Could you check a few things on this model? Use its own coordinates, in mm. A direction names the side the tool comes from. Round coordinates to 2 decimals unless told otherwise and drop trailing zeros. Order: outer loops, then holes, each group sorted by start corner. A loop starts at its lowest first (then second) coordinate and runs counter-clockwise, first axis right, second up. Notation, with made-up numbers: (44.25, 46.25) -> (54.25, 46.25) arc R7 cw to (54.25, 53.25) -> close; hole circle Ø3 at (-38.75, 37). An arc over 180 degrees is marked (long way). One line per question, with ' | ' between items.
Autodesk Inventor part; units mm, degrees
ref_plane "YZ Plane" through (0, 0, 0) normal (1, 0, 0) x (0, 1, 0)
ref_plane "XZ Plane" through (0, 0, 0) normal (0, 1, 0) x (-1, 0, 0)
ref_plane "XY Plane" through (0, 0, 0) normal (0, 0, 1) x (1, 0, 0)
sketch "Sketch1" plane through (0, 0, 0) normal (0, 0, 1) x (1, 0, 0)
  line L0 (0, -42.8392) -> (0, 0.8108)
  line L1 (0, 0) -> (49.5875, 0)
  line L2 (0, -42.8392) -> (10, -42.8392)
  line L3 (10, -42.8392) -> (49.5875, -10)
  line L4 (49.5875, -10) -> (49.5875, 0)
  line L5 (0, -42.8392) -> (0, 0)
  line L6 (0, 0) -> (49.5875, 0)
  line L7 (21.7117, 0) -> (36.5117, 0) construction
  dimension "d0" = 10
  dimension "d1" = 10
extrude "Extrusion1" add sketch "Sketch1" against normal blind 4
fillet "Fillet1" radius 2 2 edges at (49.5875, -10, -2) (10, -42.8392, -2)
sketch "Sketch2" plane through (0, 0, 0) normal (0, 0, 1) x (1, 0, 0)
  line L0 (14.6536, -1.8875) -> (0, -1.8875) construction
  line L1 (0, -1.8875) -> (0, -8.7634)
  line L2 (0, -8.7634) -> (-6.35, -8.7634)
  line L3 (-6.35, -8.7634) -> (-6.35, -14.7634)
  line L4 (-6.35, -14.7634) -> (0, -14.7634)
  line L5 (0, -14.7634) -> (0, -20.8634)
  line L6 (0, -20.8634) -> (6, -20.8634)
  line L7 (6, -20.8634) -> (6, -19.6134)
  line L8 (6, -19.6134) -> (8, -19.6134)
  line L9 (8, -19.6134) -> (8, -20.8634)
  line L10 (8, -20.8634) -> (10.65, -20.8634)
  line L11 (10.65, -20.8634) -> (10.65, -23.8634)
  line L12 (10.65, -23.8634) -> (8, -23.8634)
  line L13 (8, -23.8634) -> (8, -25.1134)
  line L14 (8, -25.1134) -> (6, -25.1134)
  line L15 (6, -25.1134) -> (6, -23.8634)
  line L16 (6, -23.8634) -> (0, -23.8634)
  line L17 (0, -23.8634) -> (0, -29.9634)
  line L18 (0, -29.9634) -> (-6.35, -29.9634)
  line L19 (-6.35, -29.9634) -> (-6.35, -35.9634)
  line L20 (-6.35, -35.9634) -> (0, -35.9634)
  line L21 (0, -35.9634) -> (0, -42.8392)
  line L22 (0, -42.8392) -> (14.6536, -42.8392)
  line L23 (14.6536, -42.8392) -> (14.6536, -1.8875) construction
  line L24 (49.5875, -14.6536) -> (49.5875, 0)
  line L25 (49.5875, 0) -> (42.7117, 0)
  line L26 (42.7117, 0) -> (42.7117, 6.35)
  line L27 (42.7117, 6.35) -> (36.7117, 6.35)
  line L28 (36.7117, 6.35) -> (36.7117, 0)
  line L29 (36.7117, 0) -> (30.6117, 0)
  line L30 (30.6117, 0) -> (30.6117, -6)
  line L31 (30.6117, -6) -> (31.8617, -6)
  line L32 (31.8617, -6) -> (31.8617, -8)
  line L33 (31.8617, -8) -> (30.6117, -8)
  line L34 (30.6117, -8) -> (30.6117, -10.65)
  line L35 (30.6117, -10.65) -> (27.6117, -10.65)
  line L36 (27.6117, -10.65) -> (27.6117, -8)
  line L37 (27.6117, -8) -> (26.3617, -8)
  line L38 (26.3617, -8) -> (26.3617, -6)
  line L39 (26.3617, -6) -> (27.6117, -6)
  line L40 (27.6117, -6) -> (27.6117, 0)
  line L41 (27.6117, 0) -> (21.5117, 0)
  line L42 (21.5117, 0) -> (21.5117, 6.35)
  line L43 (21.5117, 6.35) -> (15.5117, 6.35)
  line L44 (15.5117, 6.35) -> (15.5117, 0)
  line L45 (15.5117, 0) -> (8.6359, 0)
  line L46 (8.6359, 0) -> (8.6359, -14.6536) construction
  line L47 (8.6359, -14.6536) -> (49.5875, -14.6536) construction
  line L48 (49.5875, 0) -> (0, -42.8392)
  line L49 (8.6359, 0) -> (0, -1.8875)
  point P0 (0, 0)
extrude "Extrusion2" add sketch "Sketch2" against normal blind 4
sketch "Sketch3" plane through (0, 0, 0) normal (0, 0, 1) x (1, 0, 0)
  line L0 (14.6536, -1.8875) -> (0, -1.8875)
  line L1 (0, -1.8875) -> (0, -8.7634)
  line L2 (0, -8.7634) -> (-6.35, -8.7634)
  line L3 (-6.35, -8.7634) -> (-6.35, -14.7634)
  line L4 (-6.35, -14.7634) -> (0, -14.7634)
  line L5 (0, -14.7634) -> (0, -20.8634)
  line L6 (0, -20.8634) -> (6, -20.8634)
  line L7 (6, -20.8634) -> (6, -19.6134)
  line L8 (6, -19.6134) -> (8, -19.6134)
  line L9 (8, -19.6134) -> (8, -20.8634)
  line L10 (8, -20.8634) -> (10.65, -20.8634)
  line L11 (10.65, -20.8634) -> (10.65, -23.8634)
  line L12 (10.65, -23.8634) -> (8, -23.8634)
  line L13 (8, -23.8634) -> (8, -25.1134)
  line L14 (8, -25.1134) -> (6, -25.1134)
  line L15 (6, -25.1134) -> (6, -23.8634)
  line L16 (6, -23.8634) -> (0, -23.8634)
  line L17 (0, -23.8634) -> (0, -29.9634)
  line L18 (0, -29.9634) -> (-6.35, -29.9634)
  line L19 (-6.35, -29.9634) -> (-6.35, -35.9634)
  line L20 (-6.35, -35.9634) -> (0, -35.9634)
  line L21 (0, -35.9634) -> (0, -42.8392)
  line L22 (0, -42.8392) -> (14.6536, -42.8392)
  line L23 (14.6536, -42.8392) -> (14.6536, -1.8875)
  line L24 (49.5875, -14.6536) -> (49.5875, 0)
  line L25 (49.5875, 0) -> (42.7117, 0)
  line L26 (42.7117, 0) -> (42.7117, 6.35)
  line L27 (42.7117, 6.35) -> (36.7117, 6.35)
  line L28 (36.7117, 6.35) -> (36.7117, 0)
  line L29 (36.7117, 0) -> (30.6117, 0)
  line L30 (30.6117, 0) -> (30.6117, -6)
  line L31 (30.6117, -6) -> (31.8617, -6)
  line L32 (31.8617, -6) -> (31.8617, -8)
  line L33 (31.8617, -8) -> (30.6117, -8)
  line L34 (30.6117, -8) -> (30.6117, -10.65)
  line L35 (30.6117, -10.65) -> (27.6117, -10.65)
  line L36 (27.6117, -10.65) -> (27.6117, -8)
  line L37 (27.6117, -8) -> (26.3617, -8)
  line L38 (26.3617, -8) -> (26.3617, -6)
  line L39 (26.3617, -6) -> (27.6117, -6)
  line L40 (27.6117, -6) -> (27.6117, 0)
  line L41 (27.6117, 0) -> (21.5117, 0)
  line L42 (21.5117, 0) -> (21.5117, 6.35)
  line L43 (21.5117, 6.35) -> (15.5117, 6.35)
  line L44 (15.5117, 6.35) -> (15.5117, 0)
  line L45 (15.5117, 0) -> (8.6359, 0)
  line L46 (8.6359, 0) -> (8.6359, -14.6536)
  line L47 (8.6359, -14.6536) -> (49.5875, -14.6536)
  line L48 (0, -23.8634) -> (0, -20.8634)
  line L49 (0, -14.7634) -> (0, -29.9634)
  line L50 (27.6117, 0) -> (30.6117, 0)
  line L51 (36.7117, 0) -> (21.5117, 0)
  point P0 (0, 0)
extrude "Extrusion3" cut sketch "Sketch3" against normal blind 4 contours L6 L7 L8 L9 L10 L11 L12 L13 L14 L15 L16 L48 | L50 L30 L31 L32 L33 L34 L35 L36 L37 L38 L39 L40
sketch "Sketch4" plane through (0, 0, 0) normal (0, 0, 1) x (1, 0, 0)
  line L0 (30.6117, 0) -> (30.6117, -6)
  line L1 (30.6117, -6) -> (31.8617, -6)
  line L2 (31.8617, -6) -> (31.8617, -8)
  line L3 (31.8617, -8) -> (30.6117, -8)
  line L4 (30.6117, -8) -> (30.6117, -10.65)
  line L5 (30.6117, -10.65) -> (27.6117, -10.65)
  line L6 (27.6117, -10.65) -> (27.6117, -8)
  line L7 (27.6117, -8) -> (26.3617, -8)
  line L8 (26.3617, -8) -> (26.3617, -6)
  line L9 (26.3617, -6) -> (27.6117, -6)
  line L10 (27.6117, -6) -> (27.6117, 0)
  line L11 (27.6117, 0) -> (21.5117, 0)
  line L12 (21.5117, 0) -> (21.5117, 6.35)
  line L13 (21.5117, 6.35) -> (15.5117, 6.35)
  line L14 (15.5117, 6.35) -> (15.5117, 0)
  line L15 (15.5117, 0) -> (0, 0)
  line L16 (0, 0) -> (0, -8.7634)
  line L17 (0, -8.7634) -> (-6.35, -8.7634)
  line L18 (-6.35, -8.7634) -> (-6.35, -14.7634)
  line L19 (-6.35, -14.7634) -> (0, -14.7634)
  line L20 (0, -14.7634) -> (0, -29.9634)
  line L21 (0, -29.9634) -> (-6.35, -29.9634)
  line L22 (-6.35, -29.9634) -> (-6.35, -35.9634)
  line L23 (-6.35, -35.9634) -> (0, -35.9634)
  line L24 (0, -35.9634) -> (0, -42.8392)
  line L25 (0, -42.8392) -> (9.2784, -42.8392)
  arc A0 (9.2784, -42.8392) -> (10.5554, -42.3785) centre (9.2784, -40.8392) ccw
  line L26 (10.5554, -42.3785) -> (48.8645, -10.5998)
  arc A1 (48.8645, -10.5998) -> (49.5875, -9.0605) centre (47.5875, -9.0605) ccw
  line L27 (49.5875, -9.0605) -> (49.5875, 0)
  line L28 (49.5875, 0) -> (42.7117, 0)
  line L29 (42.7117, 0) -> (42.7117, 6.35)
  line L30 (42.7117, 6.35) -> (36.7117, 6.35)
  line L31 (36.7117, 6.35) -> (36.7117, 0)
  line L32 (36.7117, 0) -> (30.6117, 0)
  line L33 (6, -23.8634) -> (0, -23.8634)
  line L34 (0, -23.8634) -> (0, -20.8634)
  line L35 (0, -20.8634) -> (6, -20.8634)
  line L36 (6, -20.8634) -> (6, -19.6134)
  line L37 (6, -19.6134) -> (8, -19.6134)
  line L38 (8, -19.6134) -> (8, -20.8634)
  line L39 (8, -20.8634) -> (10.65, -20.8634)
  line L40 (10.65, -20.8634) -> (10.65, -23.8634)
  line L41 (10.65, -23.8634) -> (8, -23.8634)
  line L42 (8, -23.8634) -> (8, -25.1134)
  line L43 (8, -25.1134) -> (6, -25.1134)
  line L44 (6, -25.1134) -> (6, -23.8634)
  line L45 (36.7117, 0) -> (30.6117, 0)
  line L46 (27.6117, 0) -> (30.6117, 0)
  line L47 (36.9117, 0) -> (36.9117, 6.15)
  line L48 (36.9117, 6.15) -> (42.5117, 6.15)
  line L49 (42.5117, 6.15) -> (42.5117, -0.2)
  line L50 (42.5117, -0.2) -> (49.3875, -0.2)
  line L51 (49.3875, -0.2) -> (49.3875, -9.0605)
  arc A2 (48.7368, -10.4459) -> (49.3875, -9.0605) centre (47.5875, -9.0605) ccw
  line L52 (48.7368, -10.4459) -> (10.4277, -42.2246)
  arc A3 (9.2784, -42.6392) -> (10.4277, -42.2246) centre (9.2784, -40.8392) ccw
  line L53 (9.2784, -42.6392) -> (0.2, -42.6392)
  line L54 (0.2, -42.6392) -> (0.2, -35.7634)
  line L55 (0.2, -35.7634) -> (-6.15, -35.7634)
  line L56 (-6.15, -35.7634) -> (-6.15, -30.1634)
  line L57 (-6.15, -30.1634) -> (0.2, -30.1634)
  line L58 (0.2, -30.1634) -> (0.2, -14.5634)
  line L59 (0.2, -14.5634) -> (-6.15, -14.5634)
  line L60 (-6.15, -14.5634) -> (-6.15, -8.9634)
  line L61 (-6.15, -8.9634) -> (0.2, -8.9634)
  line L62 (0.2, -8.9634) -> (0.2, -0.2)
  line L63 (0.2, -0.2) -> (15.7117, -0.2)
  line L64 (15.7117, -0.2) -> (15.7117, 6.15)
  line L65 (15.7117, 6.15) -> (21.3117, 6.15)
  line L66 (21.3117, 6.15) -> (21.3117, -0.2)
  line L67 (27.4117, -0.2) -> (27.4117, -5.8)
  line L68 (27.4117, -5.8) -> (26.1617, -5.8)
  line L69 (26.1617, -5.8) -> (26.1617, -8.2)
  line L70 (26.1617, -8.2) -> (27.4117, -8.2)
  line L71 (27.4117, -8.2) -> (27.4117, -10.85)
  line L72 (27.4117, -10.85) -> (30.8117, -10.85)
  line L73 (30.8117, -10.85) -> (30.8117, -8.2)
  line L74 (30.8117, -8.2) -> (32.0617, -8.2)
  line L75 (32.0617, -8.2) -> (32.0617, -5.8)
  line L76 (32.0617, -5.8) -> (30.8117, -5.8)
  line L77 (30.8117, -5.8) -> (30.8117, 0)
  line L78 (10.85, -20.6634) -> (8.2, -20.6634)
  line L79 (8.2, -20.6634) -> (8.2, -19.4134)
  line L80 (8.2, -19.4134) -> (5.8, -19.4134)
  line L81 (5.8, -19.4134) -> (5.8, -20.6634)
  line L82 (5.8, -20.6634) -> (-0.2, -20.6634)
  line L83 (-0.2, -20.6634) -> (-0.2, -24.0634)
  line L84 (-0.2, -24.0634) -> (5.8, -24.0634)
  line L85 (5.8, -24.0634) -> (5.8, -25.3134)
  line L86 (5.8, -25.3134) -> (8.2, -25.3134)
  line L87 (8.2, -25.3134) -> (8.2, -24.0634)
  line L88 (8.2, -24.0634) -> (10.85, -24.0634)
  line L89 (10.85, -24.0634) -> (10.85, -20.6634)
  line L90 (30.8117, -0.2) -> (30.8117, 0)
  line L91 (30.8117, 0) -> (27.4117, 0)
  line L92 (27.4117, 0) -> (27.4117, -0.2)
  point P0 (0, 0)
  dimension "d9" = 0.2
  dimension "d10" = 0.2
extrude "Extrusion4" cut sketch "Sketch4" against normal blind 25.4 contours L32 L77 L76 L75 L74 L73 L72 L71 L70 L69 L68 L67 L92 L11 L10 L9 L8 L7 L6 L5 L4 L3 L2 L1 L0 | L0 L1 L2 L3 L4 L5 L6 L7 L8 L9 L10 L46 | L82 L58 L35 L20 | L20 L84 L83 L82 | L35 L58 L33 L20 | L82 L81 L80 L79 L78 L89 L88 L87 L86 L85 L84 L58 L33 L44 L43 L42 L41 L40 L39 L38 L37 L36 L35 | L33 L58 L84 L20 | L35 L36 L37 L38 L39 L40 L41 L42 L43 L44 L33 L58
sketch "Sketch5" plane through (0, 0, 0) normal (0, 0, 1) x (1, 0, 0)
  line L0 (42.9117, 4) -> (46.4125, 4)
  line L1 (-4, -102.5091) -> (-4, 2)
  line L2 (61.4276, 22.986) -> (8.4509, 22.986)
  line L3 (8.4509, 22.986) -> (8.4509, 4)
  line L4 (8.4509, 4) -> (61.4276, 4)
  line L5 (61.4276, 4) -> (61.4276, 22.986)
  line L6 (-4, 2) -> (-14.2218, 2)
  line L7 (-14.2218, 2) -> (-14.2218, -39.6128)
  line L8 (-14.2218, -39.6128) -> (-4, -39.6128)
  line L9 (-4, -39.6128) -> (-4, 2)
  point P0 (0, 0)
extrude "Extrusion5" cut sketch "Sketch5" against normal blind 25.4
fillet "Fillet2" radius 0.5 8 edges at (42.7117, 4, -2) (36.7117, 4, -2) (21.5117, 4, -2) (15.5117, 4, -2) (-4, -8.7634, -2) (-4, -14.7634, -2) (-4, -29.9634, -2) (-4, -35.9634, -2)
properties part number "motor_brace_3"
1. I want a section at B-B on y = -4.5. List the corners of the cut face in (x, z) for me, and give its area (3 significant figures).
From the geometry:
outline: (0, -4) -> (27.41, -4) -> (27.41, 0) -> (0, 0) -> close; (30.81, -4) -> (49.59, -4) -> (49.59, 0) -> (30.81, 0) -> close | area: 185 mm²
2. If we mould it in two halves opening along Y, with no side actions, what happens to faces 1 (the face through (5.8, -25, -2)), 2 (the face through (10, -20.663, -2)), 3 (the face through (15.512, 2, -2)), 4 (the face through (8, 0, -2))? For each: pulls with the +Y half, pulls with the -Y half, needs draft (parallel to the pull), parting line crosses it, or undercut.
From the geometry:
face 1: undercut | face 2: undercut | face 3: needs draft | face 4: pulls with the +Y half
3. I want a section at D-D on y = -18. List the corners of the cut face in (x, z) for me.
From the geometry:
outline: (0, -4) -> (39.94, -4) -> (39.94, 0) -> (0, 0) -> close
4. On a 3-axis mill with a long thin cutter (end or side, diameter ignored), from which of +Z, -Z, +X, -X, +Y, -Y can I reach the whole of each face in a straight line? I mean faces 5 (the face through (42.712, 2, -2)), 6 (the face through (30.812, -3, -2)), 7 (the face through (0, -4, -2)), 8 (the face through (-2, -14.763, -2)). Say none if no direction works.
From the geometry:
face 5: +Z, -Z, +X, +Y | face 6: +Z, -Z, +Y | face 7: +Z, -Z, -X, +Y | face 8: +Z, -Z, -X
5. I want a section at C-C on x = 17. List the corners of the cut face in (y, z) for me, and give its area (3 significant figures).
From the geometry:
outline: (-37.03, -4) -> (4, -4) -> (4, 0) -> (-37.03, 0) -> close | area: 164 mm²
6. I need wall thicknesses on probe 1 along X at (y, z) = (-1, -2.85); probe 2 along Y at (x, z) = (2, -0.9); probe 3 along Y at (x, z) = (-1.5, -1.8). Which ranges of each line are inside material? Lowest first, please.
From the geometry:
probe 1: x = 0 to 27.41, 30.81 to 49.59 | probe 2: y = -42.84 to -24.06, -20.66 to 0 | probe 3: y = -35.96 to -29.96, -14.76 to -8.76
7. I'm going to push flat-ended pins straight in: pin 1 (1.2 mm diameter, centred on x = 33, z = -1.5, fed in from +Y); pin 2 (1 mm diameter, centred on y = 2.5, z = -2, fed in from -X); pin 3 (1 mm diameter, centred on x = 26.5, z = -1.5, fed in from -Y). Where does each tip first touch, or does it pass through?
From the geometry:
pin 1: stops at y = 0 | pin 2: stops at x = 15.51 | pin 3: stops at y = -29.57
8. I want a section at A-A on x = 7.5. List the corners of the cut face in (y, z) for me.
From the geometry:
outline: (-42.84, -4) -> (-25.31, -4) -> (-25.31, 0) -> (-42.84, 0) -> close; (-19.41, -4) -> (0, -4) -> (0, 0) -> (-19.41, 0) -> close
